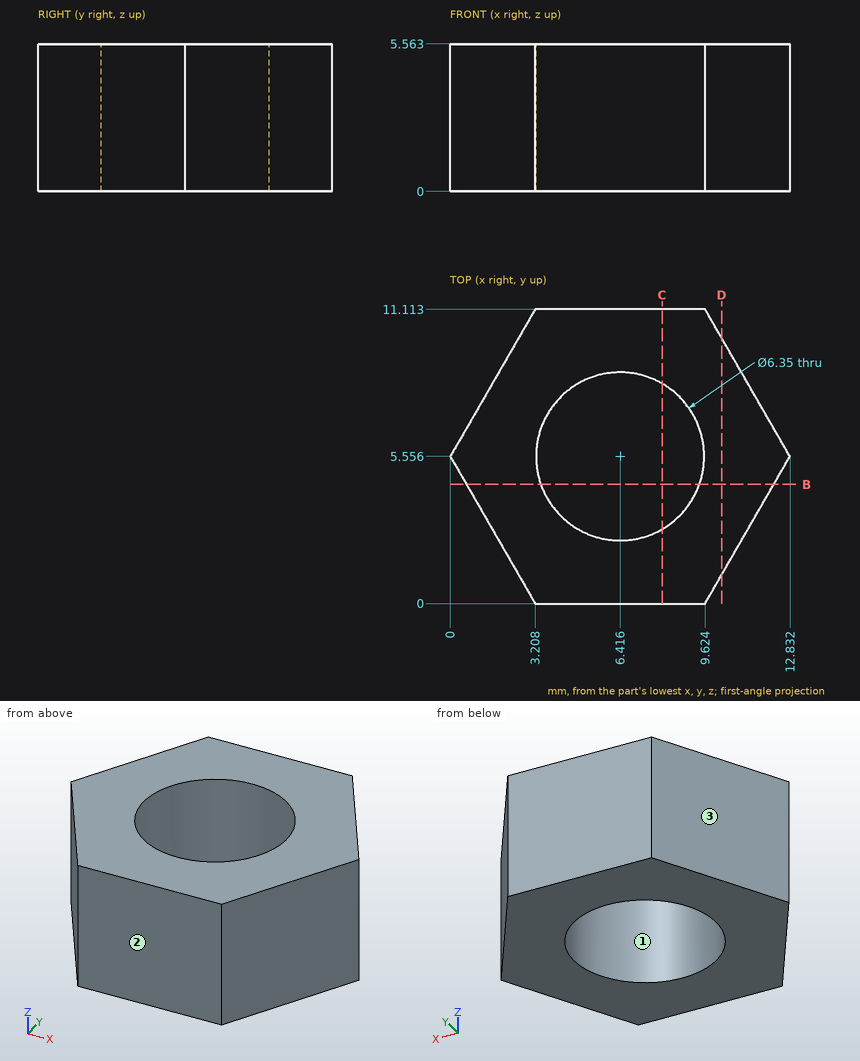
Verification items for this drawing (mm, ordinates from the low corner). Coordinates: 2 decimals unless noted, no trailing zeros. Loops run counter-clockwise (first coordinate to the right, second up) from the corner with the lowest first, then second, coordinate; pieces in that order, holes last. Notation, with made-up numbers: (55, 50) - (85, 50) arc R14 ccw to (85, 67) - close; hole circle Ø7 at (84, 66.5). An arc over 180 degrees is marked (long way). Use one line per item in the form item = value. Start each with the question number.
Item 1: Section check B-B, the plane y = 4.5. Enter the section's corners in (x, z).
Item 2: Thickness scan on probe 1 along X at (y, z) = (5.5, 5.25); probe 2 along Y at (x, z) = (5, 3.9) (1 decimal); probe 3 along X at (y, z) = (8.25, 3.35) (1 decimal). Record the ranges inside material, lowest first.
Item 3: Mould release check, pull along X, two halves, no side actions. Record for the marked faces 1, 2 and 3: +X half, -X half, draft (parallel to the pull), parting line (faces both ways), or undercut.
Item 4: Section check D-D, the plane x = 10.25. Enter the section's corners in (y, z) (1 decimal).
Item 5: Gauge pin test, flat ends, axial feed: pin 1 (1.5 mm diameter, centred on y = 5.5, z = 4.5, fed in from +X); pin 2 (3 mm diameter, centred on y = 9, z = 2.5, fed in from -X). Record the tip position at first contact, or that the pin passes through.
Item 6: Section check C-C, the plane x = 8. Enter the section's corners in (y, z) (1 decimal).
Computed:
q1.outline = (0.61, 0) - (3.42, 0) - (3.42, 5.56) - (0.61, 5.56) - close; (9.41, 0) - (12.22, 0) - (12.22, 5.56) - (9.41, 5.56) - close
q2.probe_1 = 0.03 to 3.24, 9.59 to 12.8
q2.probe_2 = 0 to 2.7, 8.4 to 11.1
q2.probe_3 = 1.6 to 4.7, 8.1 to 11.3
q3.face_1 = undercut
q3.face_2 = draft
q3.face_3 = -X half
q4.outline = (1.1, 0) - (10, 0) - (10, 5.6) - (1.1, 5.6) - close
q5.pin_1 = 12.83
q5.pin_2 = 1.12
q6.outline = (0, 0) - (2.8, 0) - (2.8, 5.6) - (0, 5.6) - close; (8.3, 0) - (11.1, 0) - (11.1, 5.6) - (8.3, 5.6) - close
